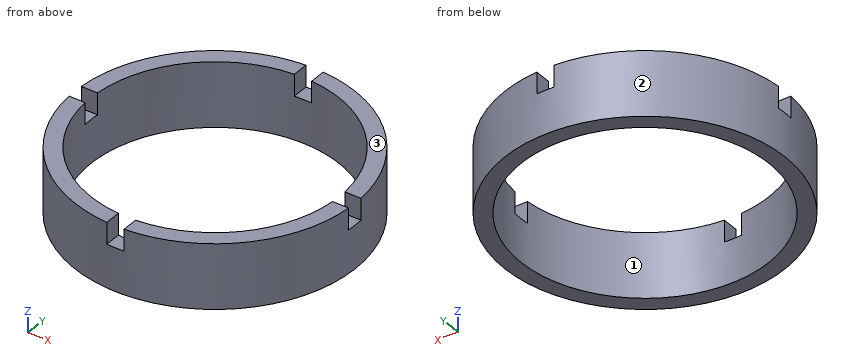
Autodesk Fusion 360 part; units mm, degrees
cylinder "CylinderPrimitive1" add diameter 65 height 15 placed x (1, 0, 0) y (0, 1, 0) z (0, 0, 1) at (0, 0, 0)
cylinder "CylinderPrimitive2" cut diameter 57.5 height -15 placed x (1, 0, 0) y (0, 1, 0) z (0, 0, 1) at (0, 0, 15)
sketch "Sketch5" plane through (0, 0, 0) normal (0, 1, 0) x (1, 0, 0)
  line L0 (0, -15) -> (0, 0)
  line L1 (-2, -15) -> (2, -15)
  line L2 (2, -15) -> (2, -10)
  line L3 (2, -10) -> (-2, -10)
  line L4 (-2, -10) -> (-2, -15)
sketch "Sketch6" plane through (0, 0, 0) normal (1, 0, 0) x (0, 1, 0)
  line L0 (0, 15) -> (0, 0)
  line L1 (-2, 15) -> (2, 15)
  line L2 (2, 15) -> (2, 10)
  line L3 (2, 10) -> (-2, 10)
  line L4 (-2, 10) -> (-2, 15)
extrude "Extrude1" cut sketch "Sketch6" along normal through all and the other way through all
extrude "Extrude2" cut sketch "Sketch5" along normal through all and the other way through all
Read the model definition and answer for the solid it produces. Units are mm, in the model's axes. Face numbers are marked on the shaded views. Coordinates: 2 decimals unless noted, no trailing zeros. Write each loop counter-clockwise with the first axis right and the second up, starting at its lowest first coordinate (ties: lowest second). Pieces come first, ordered by that corner, then holes. Notation, with made-up numbers: M 17,31.5 L 73,31.5 A31 cw 73,62.5 Z; hole C 50,-10 d5. An arc over 180 degrees is marked long. Use a Markdown table: item, result.
Q1. Each of these flat-tipped pins is pushed along its axis until it touches: pin 1 Ø1 at (y, z) = (-18.5, 5.5) entering from -X; pin 2 Ø2 at (y, z) = (-2.5, 5) entering from -X; pin 3 Ø3 at (x, y) = (-1, -30.5) entering from +Z; pin 4 Ø1.1 at (y, z) = (30.5, 12) entering from -X. Where does it stop, or does it pass through?
Answer block:
| item | result |
|---|---|
| pin 1 | stops at x = -27.06 |
| pin 2 | stops at x = -32.47 |
| pin 3 | stops at z = 15 |
| pin 4 | stops at x = -12.62 |
Q2. The part is cut by section C-C, the plane z = 11.5. Write down the section's boundary in (x, y), then the cut area to 3 significant figures.
Answer block:
| item | result |
|---|---|
| outline | M -32.44,-2 A32.5 ccw -2,-32.44 L -2,-28.68 A28.75 cw -28.68,-2 Z; M -32.44,2 L -28.68,2 A28.75 cw -2,28.68 L -2,32.44 A32.5 ccw Z; M 2,-32.44 A32.5 ccw 32.44,-2 L 28.68,-2 A28.75 cw 2,-28.68 Z; M 2,28.68 A28.75 cw 28.68,2 L 32.44,2 A32.5 ccw 2,32.44 Z |
| area | 662 mm2 |
Q3. Determine the mould class of the marked faces 1, 2 and 3 for opening direction Y: released by +Y, released by -Y, zero draft, split by the parting line, or undercut.
Answer block:
| item | result |
|---|---|
| face 1 | undercut |
| face 2 | split by the parting line |
| face 3 | zero draft |
Q4. The part is cut by section A-A, the plane y = 0. Write down the section's boundary in (x, z).
Answer block:
| item | result |
|---|---|
| outline | M -32.5,0 L -28.75,0 L -28.75,10 L -32.5,10 Z; M 28.75,0 L 32.5,0 L 32.5,10 L 28.75,10 Z |
Q5. The part is cut by section D-D, the plane z = 1. Write down the section's boundary in (x, y).
Answer block:
| item | result |
|---|---|
| outline | C 0,0 d65; hole C 0,0 d57.5 |
Q6. Straight lines are drawn through the part: L1, parallel to Y at x = 0, z = 9.25; L2, parallel to X at y = 14, z = 8.25. For each, find the intervals that lie inside material, in ascending order. Write a range as [from, to].
Answer block:
| item | result |
|---|---|
| L1 | y = [-32.5, -28.75], [28.75, 32.5] |
| L2 | x = [-29.33, -25.11], [25.11, 29.33] |
